Verification items for the finished model (mm, model axes). Give positions to 0.01 mm unless a question says otherwise; leave off trailing zeros. Loops run counter-clockwise (first coordinate to the right, second up) from the corner with the lowest first, then second, coordinate; pieces in that order, holes last. Notation, with made-up numbers: M 46,-39 L 54,-39 A19 cw 54,-6 Z; hole C 41.25,24 d8. An arc over 180 degrees is marked long. Answer in a Markdown table with one row per item.
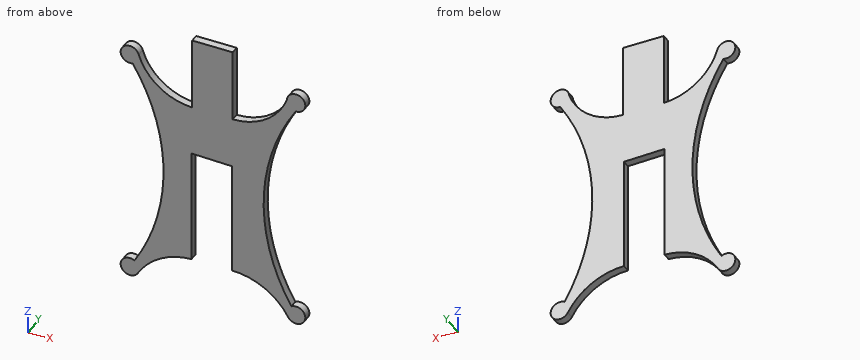
```python
from build123d import *

# Parameters (mm, degrees)
BOSS_EXTRUDE2_DEPTH = 3


with BuildPart() as part:
    # Sketch1 → Boss-Extrude2 (new body)
    with BuildSketch(Plane(origin=(0, 0, 0), x_dir=(1, 0, 0), z_dir=(0, 1, 0))):
        with BuildLine():
            Line((25.757149381, -1.351865927), (25.757149381, 41.431167148))
            ThreePointArc((25.757149381, 41.431167148), (38.075697549, 44.757926971), (47.044816732, 53.833656195))
            ThreePointArc((47.044816732, 53.833656195), (53.444849138, 52.904300859), (48.262189364, 49.035948005))
            ThreePointArc((48.262189364, 49.035948005), (37.775812363, 8.529611884), (49.927233588, -31.508748857))
            ThreePointArc((49.927233588, -31.508748857), (52.6141246, -37.391327613), (46.554594416, -35.131635139))
            ThreePointArc((46.554594416, -35.131635139), (38.575085108, -24.669898603), (26.030357143, -20.701233785))
            Line((26.030357143, -20.701233785), (26.030357143, -48.189781488))
            Line((26.030357143, -48.189781488), (10.652357143, -48.189781488))
            Line((10.652357143, -48.189781488), (10.652357143, -20.701233785))
            ThreePointArc((10.652357143, -20.701233785), (-1.954368788, -25.111263089), (-9.626768487, -36.04342573))
            ThreePointArc((-9.626768487, -36.04342573), (-16.066621017, -36.637071695), (-11.932728711, -31.663637214))
            ThreePointArc((-11.932728711, -31.663637214), (-0.214526097, 8.575081304), (-11.212333327, 49.01663143))
            ThreePointArc((-11.212333327, 49.01663143), (-16.352559443, 52.941194032), (-9.942785871, 53.800797946))
            ThreePointArc((-9.942785871, 53.800797946), (-1.352444064, 45.093210402), (10.379149381, 41.631163543))
            Line((10.379149381, 41.631163543), (10.379149381, -1.751865927))
            Line((10.379149381, -1.751865927), (25.757149381, -1.351865927))
        make_face()
    extrude(amount=BOSS_EXTRUDE2_DEPTH)


solid = part.part
```
Item 1: Scan lines: L1, parallel to X at y = 0.7, z = 27; L2, parallel to X at y = 1.95, z = 24.5; L3, parallel to Z at x = 49.5, y = 0.1. Record each from-to range of solid material in increasing order. Write a range as [from, to].
Reported:
| item | result |
|---|---|
| L1 | x = [-9.24, -4.13], [10.65, 26.03], [41.36, 47.26] |
| L2 | x = [-7.97, -1.1], [10.65, 26.03], [38.33, 45.95] |
| L3 | z = [-55.5, -48.59], [30.83, 38.46] |
Item 2: Sectioned sample at B-B (z = -24.5). Record the cut outline in (x, y), and give its area (3 significant figures).
Reported:
| item | result |
|---|---|
| outline | M -1.73,0 L 10.38,0 L 10.38,3 L -1.73,3 Z; M 25.76,0 L 39.11,0 L 39.11,3 L 25.76,3 Z |
| area | 76.4 mm^2 |
Item 3: Sectioned sample at C-C (z = 34). Record the cut outline in (x, y).
Reported:
| item | result |
|---|---|
| outline | M -16.32,0 L -8.88,0 L -8.88,3 L -16.32,3 Z; M 10.65,0 L 26.03,0 L 26.03,3 L 10.65,3 Z; M 46.11,0 L 53.4,0 L 53.4,3 L 46.11,3 Z |
Item 4: Sectioned sample at A-A (x = -3). Record the cut outline in (y, z), and give its area (3 significant figures).
Reported:
| item | result |
|---|---|
| outline | M 0,-46.17 L 3,-46.17 L 3,-29.84 L 0,-29.84 Z; M 0,11.31 L 3,11.31 L 3,25.95 L 0,25.95 Z |
| area | 92.9 mm^2 |
Item 5: Sectioned sample at D-D (y = 1.45). Record the cut outline in (x, z) (3 decimals).
Reported:
| item | result |
|---|---|
| outline | M -11.933,31.664 A77.32 cw -11.212,-49.017 A3.5 ccw long -9.943,-53.801 A24.47 cw 10.379,-41.631 L 10.379,1.752 L 25.757,1.352 L 25.757,-41.431 A24.47 cw 47.045,-53.834 A3.5 ccw long 48.262,-49.036 A77.32 cw 49.927,31.509 A3.5 ccw long 46.555,35.132 A21.811 cw 26.03,20.701 L 26.03,48.19 L 10.652,48.19 L 10.652,20.701 A21.811 cw -9.627,36.043 A3.5 ccw long Z |
Item 6: Go/stop test with flat-tipped pins: pin 1 (1.5 mm diameter, centred on y = 1, z = -25.5, fed in from -X); pin 2 (1 mm diameter, centred on y = 2, z = -40, fed in from -X). Record where each tip stops, or that it passes through.
Reported:
| item | result |
|---|---|
| pin 1 | stops at x = -2.1 |
| pin 2 | stops at x = -6.8 |
